CAD build for the part. Positions are in the model's coordinates, mm. A direction names the side the tool comes from. Give positions to 0.01 mm unless a question says otherwise; leave off trailing zeros. Loops run counter-clockwise (first coordinate to the right, second up) from the corner with the lowest first, then second, coordinate; pieces in that order, holes last. Notation, with made-up numbers: M 14,43.25 L 36,43.25 A10 ccw 36,61.25 Z; hole C 2.5,42.25 d7. An arc over 180 degrees is marked long. One line per question, with ' | ' between items.
Autodesk Inventor part; units mm, degrees
ref_plane "YZ Plane" through (0, 0, 0) normal (1, 0, 0) x (0, 1, 0)
ref_plane "XZ Plane" through (0, 0, 0) normal (0, 1, 0) x (-1, 0, 0)
ref_plane "XY Plane" through (0, 0, 0) normal (0, 0, 1) x (1, 0, 0)
sketch "Sketch1" plane through (0, 0, 0) normal (0, 1, 0) x (-1, 0, 0)
  line L0 (21.5102, 17.7267) -> (21.5102, -43.9733)
  line L1 (21.5102, -43.9733) -> (19.1102, -46.7733)
  line L2 (19.1102, -46.7733) -> (-5.4898, -46.7733)
  line L3 (-5.4898, -46.7733) -> (-7.4898, -44.7733)
  line L4 (-7.4898, -44.7733) -> (-7.4898, 9.2267)
  line L5 (-7.4898, 9.2267) -> (5.5102, 22.2267)
  line L6 (5.5102, 22.2267) -> (17.0102, 22.2267)
  line L7 (17.0102, 22.2267) -> (21.5102, 17.7267)
  line L8 (22.0102, 21.7267) -> (22.0102, -46.2733)
  line L9 (22.0102, -46.2733) -> (21.0102, -47.2733)
  line L10 (21.0102, -47.2733) -> (-6.9898, -47.2733)
  line L11 (-6.9898, -47.2733) -> (-7.9898, -46.2733)
  line L12 (-7.9898, -46.2733) -> (-7.9898, 9.7267)
  line L13 (-7.9898, 9.7267) -> (5.0102, 22.7267)
  line L14 (5.0102, 22.7267) -> (21.0102, 22.7267)
  line L15 (21.0102, 22.7267) -> (22.0102, 21.7267)
  point P0 (0, 0)
  point P1 (14.1019, -14.4492)
  dimension "d0" = 69
  dimension "d1" = 29
  dimension "d2" = 2
  dimension "d3" = 2
  dimension "d4" = 2.8
  dimension "d5" = 2.4
  dimension "d6" = 4.5
  dimension "d7" = 4.5
  dimension "d8" = 13
  dimension "d9" = 13
  dimension "d10" = 70
  dimension "d11" = 30
  dimension "d12" = 1
  dimension "d13" = 1
  dimension "d14" = 1
  dimension "d15" = 1
  dimension "d16" = 1
  dimension "d17" = 1
  dimension "d18" = 13
  dimension "d19" = 13
  dimension "d34" = 0.5
  dimension "d35" = 0.5
extrude "Extrusion1" add sketch "Sketch1" along normal blind 0.5 contours L0 L1 L2 L3 L4 L5 L6 L7 | L8 L9 L10 L11 L12 L13 L14 L15
extrude "Extrusion2" add sketch "Sketch1" along normal blind 9.2
sketch "Sketch2" plane through (0, 0.5, 0) normal (0, 1, 0) x (1, 0, 0)
  circle A0 centre (-20.6484, -17.3121) radius 0.5
  circle A1 centre (-16.6313, -21.3691) radius 0.5
  circle A2 centre (-5.7074, -21.3691) radius 0.5
  circle A3 centre (6.7103, -8.921) radius 0.5
  circle A4 centre (6.7103, 44.2469) radius 0.5
  circle A5 centre (5.3281, 46.0012) radius 0.5
  circle A6 centre (-20.6484, 43.7469) radius 0.5
  circle A7 centre (-18.7007, 46.0012) radius 0.5
  point P0 (0, 0)
  dimension "d24" = 1
  dimension "d25" = 1
  dimension "d26" = 1
  dimension "d27" = 1
  dimension "d28" = 1
  dimension "d29" = 1
  dimension "d30" = 1
  dimension "d31" = 1
extrude "Extrusion3" add sketch "Sketch2" along normal blind 1.4
sketch "Sketch3" plane through (0, 9.2, 0) normal (0, 1, 0) x (1, 0, 0)
  line L0 (-21.0102, -22.7267) -> (-5.0102, -22.7267)
  line L1 (-5.0102, -22.7267) -> (7.9898, -9.7267)
  line L2 (7.9898, -9.7267) -> (7.9898, 46.2733)
  line L3 (7.9898, 46.2733) -> (6.9898, 47.2733)
  line L4 (6.9898, 47.2733) -> (-21.0102, 47.2733)
  line L5 (-21.0102, 47.2733) -> (-22.0102, 46.2733)
  line L6 (-22.0102, 46.2733) -> (-22.0102, -21.7267)
  line L7 (-22.0102, -21.7267) -> (-21.0102, -22.7267)
  line L8 (-21.5102, -17.7267) -> (-21.5102, 43.9733)
  line L9 (-19.1102, 46.7733) -> (5.4898, 46.7733)
  line L10 (7.4898, 44.7733) -> (7.4898, -9.2267)
  line L11 (7.4898, -9.2267) -> (-5.5102, -22.2267)
  line L12 (-5.5102, -22.2267) -> (-17.0102, -22.2267)
  line L13 (-17.0102, -22.2267) -> (-21.5102, -17.7267)
  line L14 (-5.5102, -22.2267) -> (-17.0102, -22.2267)
  line L15 (-21.0102, -22.7267) -> (-5.0102, -22.7267)
  line L16 (-16.0102, -22.2267) -> (-6.9102, -22.2267)
  line L17 (-6.9102, -22.2267) -> (-6.9102, -22.7267)
  line L18 (-6.9102, -22.7267) -> (-16.0102, -22.7267)
  line L19 (-16.0102, -22.7267) -> (-16.0102, -22.2267)
  line L20 (-21.5102, 43.9733) -> (-19.1102, 46.7733)
  line L21 (5.4898, 46.7733) -> (7.4898, 44.7733)
  line L22 (7.4898, -4.7267) -> (7.9898, -4.7267)
  line L23 (7.9898, -4.7267) -> (7.9898, 4.3733)
  line L24 (7.9898, 4.3733) -> (7.4898, 4.3733)
  line L25 (7.4898, 4.3733) -> (7.4898, -4.7267)
  line L26 (7.4898, 10.2733) -> (7.9898, 10.2733)
  line L27 (7.9898, 10.2733) -> (7.9898, 19.3733)
  line L28 (7.9898, 19.3733) -> (7.4898, 19.3733)
  line L29 (7.4898, 19.3733) -> (7.4898, 10.2733)
  line L30 (7.4898, 25.1733) -> (7.9898, 25.1733)
  line L31 (7.9898, 25.1733) -> (7.9898, 38.3733)
  line L32 (7.9898, 38.3733) -> (7.4898, 38.3733)
  line L33 (7.4898, 38.3733) -> (7.4898, 25.1733)
  line L34 (-22.0102, -6.8267) -> (-21.5102, -6.8267)
  line L35 (-21.5102, -6.8267) -> (-21.5102, 6.3733)
  line L36 (-21.5102, 6.3733) -> (-22.0102, 6.3733)
  line L37 (-22.0102, 6.3733) -> (-22.0102, -6.8267)
  line L38 (-21.5102, 43.9733) -> (-21.5102, -17.7267)
  line L39 (-22.0102, 9.6733) -> (-21.5102, 9.6733)
  line L40 (-21.5102, 9.6733) -> (-21.5102, 22.8733)
  line L41 (-21.5102, 22.8733) -> (-22.0102, 22.8733)
  line L42 (-22.0102, 22.8733) -> (-22.0102, 9.6733)
  line L43 (-22.0102, 25.1733) -> (-21.5102, 25.1733)
  line L44 (-21.5102, 25.1733) -> (-21.5102, 38.3733)
  line L45 (-21.5102, 38.3733) -> (-22.0102, 38.3733)
  line L46 (-22.0102, 38.3733) -> (-22.0102, 25.1733)
  point P0 (0, 0)
  point P1 (-16.0102, -22.4767)
  point P2 (-6.9102, -22.4767)
  point P3 (7.7398, -4.7267)
  point P4 (7.7398, 4.3733)
  point P5 (7.7398, 19.3733)
  point P6 (7.7398, 10.2733)
  point P7 (7.7398, 25.1733)
  point P8 (7.7398, 38.3733)
  point P9 (-21.7602, 6.3733)
  point P10 (-21.7602, -6.8267)
  point P11 (-21.7602, 9.6733)
  point P12 (-21.7602, 22.8733)
  point P13 (-21.7602, 38.3733)
  point P14 (-21.7602, 25.1733)
  dimension "d36" = 1
  dimension "d37" = 1.4
  dimension "d38" = 4.5
  dimension "d39" = 9.1
  dimension "d40" = 5.7462
  dimension "d41" = 5.9
  dimension "d42" = 9.1
  dimension "d43" = 5.8
  dimension "d44" = 13.2
  dimension "d45" = 13.2
  dimension "d46" = 10.9
  dimension "d47" = 3.3
  dimension "d48" = 13.2
  dimension "d49" = 13.2
  dimension "d50" = 2.3
extrude "Extrusion4" cut sketch "Sketch3" against normal blind 5.7 contours L19 L12 L17 L0 | L6 L36 L8 L34 | L6 L41 L8 L39 | L22 L10 L24 L2 | L6 L45 L8 L43 | L26 L10 L28 L2 | L30 L10 L32 L2
sketch "Sketch4" plane through (0, 9.2, 0) normal (0, 1, 0) x (1, 0, 0)
  line L0 (-6.9102, -22.7267) -> (-16.0102, -22.7267)
  line L1 (-6.9102, -22.2267) -> (-6.9102, -22.7267)
  line L2 (-16.0102, -22.2267) -> (-6.9102, -22.2267)
  line L3 (-16.0102, -22.7267) -> (-16.0102, -22.2267)
  line L4 (7.4898, -4.7267) -> (7.4898, 4.3733)
  line L5 (7.9898, -4.7267) -> (7.4898, -4.7267)
  line L6 (7.9898, 4.3733) -> (7.9898, -4.7267)
  line L7 (7.4898, 4.3733) -> (7.9898, 4.3733)
  line L8 (7.4898, 10.2733) -> (7.4898, 19.3733)
  line L9 (7.9898, 10.2733) -> (7.4898, 10.2733)
  line L10 (7.9898, 19.3733) -> (7.9898, 10.2733)
  line L11 (7.4898, 19.3733) -> (7.9898, 19.3733)
  point P0 (0, 0)
extrude "Extrusion5" add sketch "Sketch4" against normal blind 2.54
sketch "Sketch5" plane through (0, 9.2, 0) normal (0, 1, 0) x (1, 0, 0)
  circle A0 centre (-20.3864, -20.9025) radius 1
  circle A1 centre (-20.8742, 46.0372) radius 0.5
  circle A2 centre (7.0371, 46.2575) radius 0.5
  point P0 (0, 0)
  dimension "d55" = 2
  dimension "d56" = 1
  dimension "d57" = 1
extrude "Extrusion6" add sketch "Sketch5" along normal blind 3.175
equation "\"d9\" = d8"
equation "\"d19\" = d18"
properties part number "Bottom"
Item 1: Drill centre lines: line 1 along X through (y, z) = (3, -39.5); line 2 along Z through (x, y) = (-12.5, 0.75); line 3 along Y through (x, z) = (-19, -35.5). Where is each one in solid material? Low to high. Write a range as [from, to].
Conclusion:
line 1: [-22.01, -21.51], [7.49, 7.99] | line 2: [-47.27, -46.77], [22.23, 22.73] | line 3: [0, 0.5]
Item 2: Saw through at B-B on y = 8.25. State how many separate pieces and enclosed holes the cut face has, and give its area (3 significant figures).
Conclusion:
separate pieces: 4 | enclosed holes: 0 | area: 86.6 mm²
Item 3: Saw through at D-D on z = -34. Give the cut face in (x, y), and give its area (3 significant figures).
Conclusion:
outline: M -22.01,0 L 7.99,0 L 7.99,3.5 L 7.49,3.5 L 7.49,0.5 L -21.51,0.5 L -21.51,3.5 L -22.01,3.5 Z | area: 18.0 mm²
Item 4: 3-axis set-ups, long thin cutter, end or side, ignore diameter. For faces 1 (the flat face through (-7, 0, -12)), 2 (the cylindrical face through (-21.12, 10.77, 21.58)): which of +Z, -Z, +X, -X, +Y, -Y reach the whole face in a straight line?
Conclusion:
face 1: +Z, -Z, +X, -X, -Y | face 2: +Y
Item 5: Mould opens along X. For faces 3 (the flat face through (-22.01, 2, -12)), 4 (the flat face through (-13, 2, 22.727)), 5 (the flat face through (7.99, 2, -19)), 6 (the flat face through (-21.51, 3, -13)) say: pulls with the +X half, pulls with the -X half, needs draft (parallel to the pull), parting line crosses it, or undercut.
Conclusion:
face 3: pulls with the -X half | face 4: needs draft | face 5: pulls with the +X half | face 6: undercut
Item 6: Saw through at A-A on z = 2. Give the cut face in (x, y), and give its area (3 significant figures).
Conclusion:
outline: M -22.01,0 L 7.99,0 L 7.99,3.5 L 7.49,3.5 L 7.49,0.5 L -21.51,0.5 L -21.51,3.5 L -22.01,3.5 Z; M 7.49,6.66 L 7.99,6.66 L 7.99,9.2 L 7.49,9.2 Z | area: 19.3 mm²
Item 7: Saw through at C-C on y = 2.75. Give the cut face in (x, z), and give its area (3 significant figures).
Conclusion:
outline: M -22.01,-46.27 L -21.01,-47.27 L 6.99,-47.27 L 7.99,-46.27 L 7.99,9.73 L -5.01,22.73 L -21.01,22.73 L -22.01,21.73 Z; hole M -21.51,-43.97 L -19.11,-46.77 L 5.49,-46.77 L 7.49,-44.77 L 7.49,9.23 L -5.51,22.23 L -17.01,22.23 L -21.51,17.73 Z | area: 113 mm²
Item 8: Drop a flat-ended pin along its axis: P1, Ø0.8, axis at x = -18.5, z = -46, coming from the +Y side. Give the stop position or say it passes through.
Conclusion:
P1: y = 1.9
